Drawing for the job (mm, zero at the part's lowest x, y, z). A direction names the side the tool comes from. Give positions to 0.01 mm unless a question says otherwise; leave off trailing zeros. Write each loop counter-clockwise with the first axis right and the second up, starting at its lowest first coordinate (ties: lowest second). Pieces come first, ordered by that corner, then holes. Notation, with made-up numbers: M 40.5,13.5 L 49.5,13.5 A12 cw 49.5,36.5 Z; hole C 88.25,86.5 d9. An arc over 180 degrees is marked long. Use CSV: the item, a comma, the result in double quotes. Start each with the question number.
1. Drill centre lines: line 1 along Y through (x, z) = (0.65, 1.9); line 2 along Z through (x, y) = (2.4, 5.5) (1 decimal); line 3 along Z through (x, y) = (1.3, 3) (1 decimal). Where is each one in solid material? Low to high. Write a range as from..to.
2. Band-saw the part on A-A, the plane x = 2.15. List the corners of the cut face in (y, z).
3. 3-axis set-ups, long thin cutter, end or side, ignore diameter. For the marked faces 1 and 2: which of +Z, -Z, +X, -X, +Y, -Y reach the whole face in a straight line?
4. Band-saw the part on B-B, the plane z = 2.15. List the corners of the cut face in (x, y).
5. Drop a flat-ended pin along its axis: pin 1 Ø1.5 at (x, y) = (2.5, 5.5) entering from +Z. Give the stop position or say it passes through.
6. Band-saw the part on C-C, the plane y = 7.75. List the corners of the cut face in (x, z).
7. Band-saw the part on D-D, the plane z = 0.75. List the corners of the cut face in (x, y).
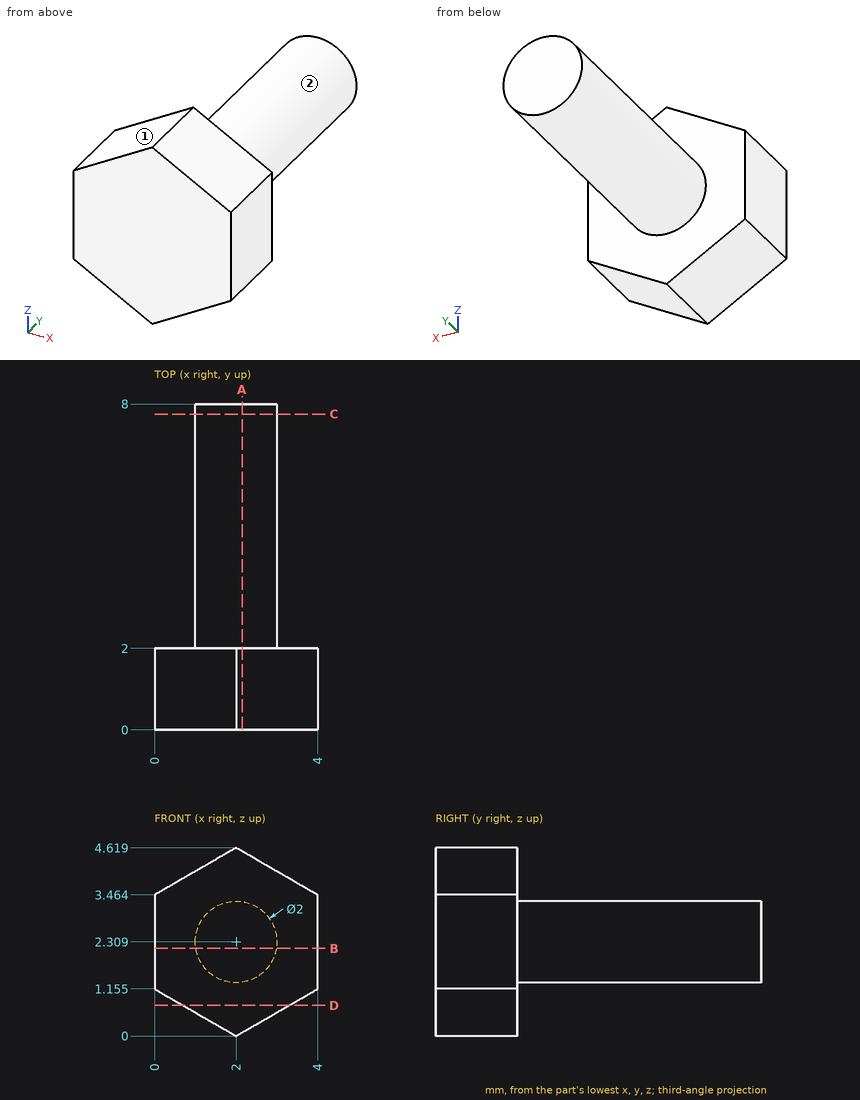
Output:
1,line 1,"y = 0..2"
1,line 2,"z = 1.4..3.2"
1,line 3,"z = 1.6..3"
2,outline,"M 0,0.09 L 2,0.09 L 2,1.32 L 8,1.32 L 8,3.3 L 2,3.3 L 2,4.53 L 0,4.53 Z"
3,face 1,"+Z, -X, +Y, -Y"
3,face 2,"+Y"
4,outline,"M 0,0 L 4,0 L 4,2 L 2.99,2 L 2.99,8 L 1.01,8 L 1.01,2 L 0,2 Z"
5,pin 1,"stops at z = 3.31"
6,outline,"C 2,2.31 d2"
7,outline,"M 0.7,0 L 3.3,0 L 3.3,2 L 0.7,2 Z"
